from build123d import *

# Parameters (mm, degrees)
F0_W     = 1.5
F0_H     = 5
F1_DEPTH = 10


with BuildPart() as f1:
    # F0 (on Front) → F1 (new body)
    with BuildSketch(Plane.XZ):
        with BuildLine():
            Line((10, -10), (10, 0))
            ThreePointArc((10, 0), (0, 10), (-10, 0))
            Line((-10, 0), (-10, -10))
            Line((-10, -10), (-8.5, -10))
            Line((-8.5, -10), (-8.5, 0))
            ThreePointArc((-8.5, 0), (0, 8.5), (8.5, 0))
            Line((8.5, 0), (8.5, -10))
            Line((8.5, -10), (10, -10))
        make_face()
        with Locations((9.25, -12.5)):
            Rectangle(F0_W, F0_H)
        with Locations((-9.25, -12.5)):
            Rectangle(F0_W, F0_H)
    extrude(amount=F1_DEPTH)


solid = f1.part
CAD build for the part. Positions are in the model's coordinates, mm. A direction names the side the tool comes from. Give positions to 0.01 mm unless a question says otherwise; leave off trailing zeros. Write each loop counter-clockwise with the first axis right and the second up, starting at its lowest first coordinate (ties: lowest second). Pieces come first, ordered by that corner, then holes. Notation, with made-up numbers: M 0.25,55.25 L 32.25,55.25 A10 cw 32.25,63.25 Z; hole C -20,-25 d5. An arc over 180 degrees is marked long. Put each result on its own line as item: value. Start each with the question number.
(1) Which spindle directions (+Z, -Z, +X, -X, +Y, -Y) get a long thin tool onto all of the face, cutting with end or side? Do faces 5 (the face through (-9, -5, -15)), 6 (the face through (-8.5, -5, -8)). Say none if no direction does.
(2) Flat gauge pins, fed straight in: pin 1 Ø6 at (y, z) = (-8.5, 0.5) entering from +X; pin 2 Ø2 at (y, z) = (-7.5, 7) entering from -X; pin 3 Ø4 at (x, y) = (2.5, -4.5) entering from -Z. Where does each tip first touch, or does it go through?
(3) Band-saw the part on D-D, the plane z = -13.5. Write the cut outline in (x, y), and give its area (3 significant figures).
(4) Mould opens along X. For faces 1 (the face through (10, -5, -8)), 2 (the face through (-9, -10, -2)), 3 (the face through (0, -5, 10)), 4 (the face through (8.5, -5, -7)) say: +X half, -X half, draft (parallel to the pull), parting line (faces both ways), or undercut.
(5) Band-saw the part on B-B, the plane y = -8.5. Write the cut outline in (x, z), and give its area (3 significant figures).
(6) Band-saw the part on A-A, the plane z = 4.25. Write the cut outline in (x, y), and give its area (3 significant figures).
(7) Probe L1, parallel to X at y = -2, z = -7.75; L2, parallel to X at y = -2.75, z = 4.75; L3, parallel to Z at x = 0.25, y = -9.5. List the from-to ranges inside material, lowest first.
(8) Band-saw the part on C-C, the plane x = 0. Write the cut outline in (y, z), and give its area (3 significant figures).
Response values:
1. face 5: -Z, +X, -X, +Y, -Y
1. face 6: -Z, +Y, -Y
2. pin 1: stops at x = 10
2. pin 2: stops at x = -8
2. pin 3: stops at z = 7.21
3. outline: M -10,-10 L -8.5,-10 L -8.5,0 L -10,0 Z; M 8.5,-10 L 10,-10 L 10,0 L 8.5,0 Z
3. area: 30.0 mm2
4. face 1: +X half
4. face 2: draft
4. face 3: parting line
4. face 4: undercut
5. outline: M -10,-15 L -8.5,-15 L -8.5,0 A8.5 cw 8.5,0 L 8.5,-15 L 10,-15 L 10,0 A10 ccw -10,0 Z
5. area: 88.6 mm2
6. outline: M -9.05,-10 L -7.36,-10 L -7.36,0 L -9.05,0 Z; M 7.36,-10 L 9.05,-10 L 9.05,0 L 7.36,0 Z
6. area: 33.8 mm2
7. L1: x = -10 to -8.5, 8.5 to 10
7. L2: x = -8.8 to -7.05, 7.05 to 8.8
7. L3: z = 8.5 to 10
8. outline: M -10,8.5 L 0,8.5 L 0,10 L -10,10 Z
8. area: 15.0 mm2
